Could you check a few things on this model? Use its own coordinates, in mm. Round coordinates to 2 decimals unless told otherwise and drop trailing zeros. Write each loop counter-clockwise with the first axis right and the second up, starting at its lowest first coordinate (ties: lowest second). Pieces come first, ordered by that corner, then holes. Notation, with made-up numbers: (51, -8.75) -> (85, -8.75) arc R20 cw to (85, 10.25) -> close; hole circle Ø5 at (-12, 28.25). An arc over 180 degrees is marked (long way). Answer as CSV lines item,"result". Start each with the question number.
Q1. If I drill on line 1 (Y direction, x = -103, z = -11); line 2 (Z direction, x = -448.5, y = -7.5); line 3 (Y direction, x = -488.5, z = 0.75), over which ranges is the centre line in solid material (lowest first)? Write a range as [from, to].
Q2. Imagine slicing it at B-B on y = -4. Please give me the cut outline in (x, z).
Q3. Will this pin go through, and if not, where does the flat tip stop? pin 1 Ø1.5 at (x, y) = (-262.5, 4.5) entering from -Z.
Q4. Imagine slicing it at A-A on x = 292. Please give me the cut outline in (y, z).
from build123d import *

# Parameters (mm, degrees)
F1_DEPTH = 1270
F2_W     = 1143
F2_H     = 13.208
F3_DEPTH = 1270


with BuildPart() as f1:
    # F0 (on Right) → F1 (new body, symmetric)
    with BuildSketch(Plane.YZ):
        with BuildLine():
            ThreePointArc((-7.9375, 1.524), (-9.015131, 1.077631), (-9.4615, 0))
            Line((-9.4615, 0), (-9.4615, -11.684))
            Line((-9.4615, -11.684), (-7.9375, -11.684))
            Line((-7.9375, -11.684), (-7.9375, 0))
            Line((-7.9375, 0), (7.9375, 0))
            Line((7.9375, 0), (7.9375, -11.684))
            Line((7.9375, -11.684), (9.4615, -11.684))
            Line((9.4615, -11.684), (9.4615, 0))
            ThreePointArc((9.4615, 0), (9.015131, 1.077631), (7.9375, 1.524))
            Line((7.9375, 1.524), (-7.9375, 1.524))
        make_face()
    extrude(amount=F1_DEPTH, both=True)

    # F2 (on Front) → F3 (intersect, symmetric)
    with BuildSketch(Plane.XZ):
        with Locations((0, -5.08)):
            Rectangle(F2_W, F2_H)
    extrude(amount=F3_DEPTH, both=True, mode=Mode.INTERSECT)


solid = f1.part
Checks:
1,line 1,"[-9.46, -7.94], [7.94, 9.46]"
1,line 2,"[0, 1.52]"
1,line 3,"[-9.26, 9.26]"
2,outline,"(-571.5, 0) -> (571.5, 0) -> (571.5, 1.52) -> (-571.5, 1.52) -> close"
3,pin 1,"z = 0"
4,outline,"(-9.46, -11.68) -> (-7.94, -11.68) -> (-7.94, 0) -> (7.94, 0) -> (7.94, -11.68) -> (9.46, -11.68) -> (9.46, 0) arc R1.52 ccw to (7.94, 1.52) -> (-7.94, 1.52) arc R1.52 ccw to (-9.46, 0) -> close"
